Read the model definition and answer for the solid it produces. Units are mm, in the model's axes. Face numbers are marked on the shaded views. Round coordinates to 2 decimals unless told otherwise and drop trailing zeros. Write each loop counter-clockwise with the first axis right and the second up, starting at its lowest first coordinate (ties: lowest second). Pieces come first, ordered by that corner, then holes.
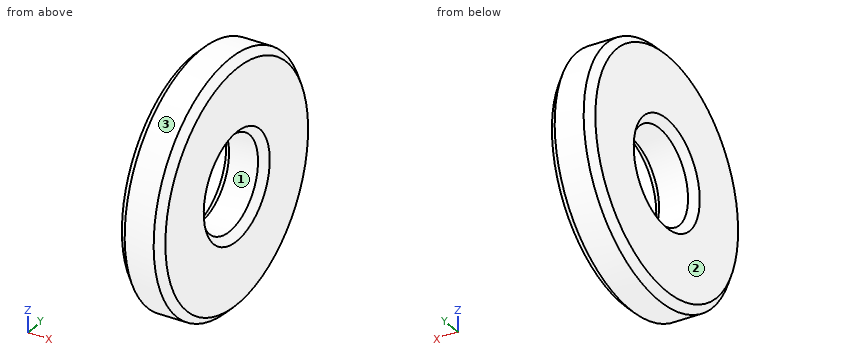
from build123d import *

# Parameters (mm, degrees)
ESQUISSE1_W     = 3
ESQUISSE1_H     = 5.3
CHANFREIN1_SIZE = 0.5


with BuildPart() as part:
    # Esquisse1 → Base-Révolution (revolve)
    with BuildSketch(Plane.XY, mode=Mode.PRIVATE) as base_r_volution_sk:
        with Locations((1.5, 5.85)):
            Rectangle(ESQUISSE1_W, ESQUISSE1_H)
    revolve(base_r_volution_sk.sketch.rotate(Axis((0, 0, 0), (1, 0, 0)), 90), axis=Axis((0, 0, 0), (1, 0, 0)))

    # Chanfrein1
    chanfrein1_edges = [part.edges().sort_by_distance(p)[0] for p in [
        (0, 0, -3.2),
        (3, 0, -3.2),
        (3, 0, -8.5),
        (0, 0, -8.5),
    ]]
    chamfer(chanfrein1_edges, length=CHANFREIN1_SIZE)


solid = part.part
Q1. Section C-C (x = 0.8) is taken. Determine the outline of the cut face in (y, z), then the cut area to 3 significant figures.
Verdict:
outline: circle Ø17 at (0, 0); hole circle Ø6.4 at (0, 0)
area: 195 mm2
Q2. Section A-A (y = 0) is taken. Determine the outline of the cut face in (x, z), then the cut area to 3 significant figures.
Verdict:
outline: (0, -8) - (0.5, -8.5) - (2.5, -8.5) - (3, -8) - (3, -3.7) - (2.5, -3.2) - (0.5, -3.2) - (0, -3.7) - close; (0, 3.7) - (0.5, 3.2) - (2.5, 3.2) - (3, 3.7) - (3, 8) - (2.5, 8.5) - (0.5, 8.5) - (0, 8) - close
area: 30.8 mm2
Q3. Determine the mould class of the marked faces 1, 2 and 3 for opening direction Y: pulls with the +Y half, pulls with the -Y half, needs draft (parallel to the pull), parting line crosses it, or undercut.
Verdict:
face 1: undercut
face 2: needs draft
face 3: parting line crosses it
Q4. Straight lines are drawn through the part: probe 1 along Y at (x, z) = (1.2, 0); probe 2 along Y at (x, z) = (2.25, -2.25); probe 3 along Z at (x, y) = (2.45, -6). For each, find the intervals that lie inside material, in ascending order.
Verdict:
probe 1: y = -8.5 to -3.2, 3.2 to 8.5
probe 2: y = -8.2 to -2.28, 2.28 to 8.2
probe 3: z = -6.02 to 6.02
